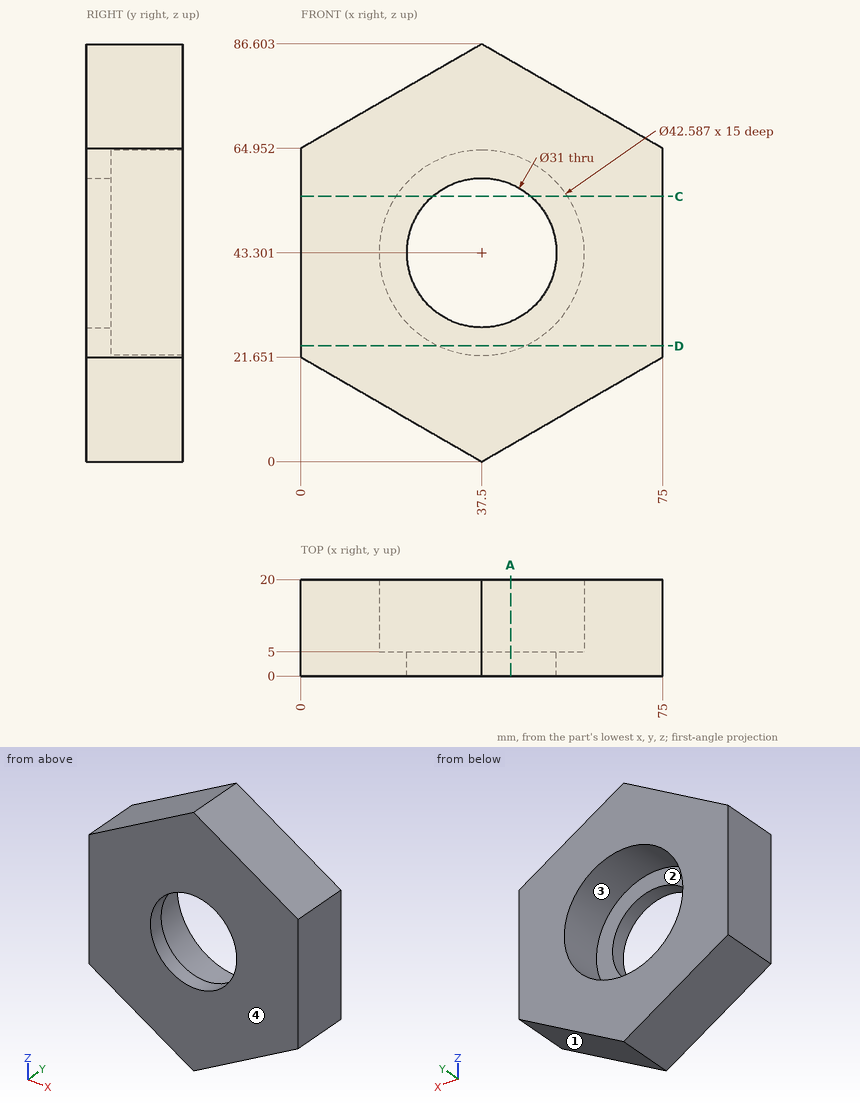
Design review of the part shown in the three views and the two pictorial views. Dimensions are in mm from the part's minimum x, y and z. Coordinates: 2 decimals unless noted, no trailing zeros. Loops run counter-clockwise (first coordinate to the right, second up) from the corner with the lowest first, then second, coordinate; pieces in that order, holes last. Notation, with made-up numbers: (-20.75, 79.25) - (37.25, 79.25) arc R24 cw to (37.25, 113.25) - close; hole circle Ø3 at (40.25, 27). An arc over 180 degrees is marked (long way). Use a Markdown table: item, result. Add a question column.
Item 1: Mouldability with a two-part tool opening along Z and no side actions: class the marked faces 1, 2, 3 and 4 as pulls with the +Z half, pulls with the -Z half, needs draft (parallel to the pull), parting line crosses it, or undercut.
Item 2: For line 1 (Z direction, x = 20, y = 9.5) (1 decimal); line 2 (Z direction, x = 33, y = 7) (1 decimal); line 3 (X direction, y = 8.25, z = 26) (1 decimal), list the stretches that pass through material, from the lowest coordinate up.
Item 3: Insertion check: pin 1 Ø1 at (x, y) = (30, 10) entering from +Z; pin 2 Ø1.5 at (x, y) = (35.5, 10.5) entering from -Z; pin 3 Ø21.5 at (x, z) = (43, 49.5) entering from +Y. Each pin has a flat end and moves straight along its axis. Give the tip position at first contact, or say it passes through.
Item 4: We need section D-D (z = 24). Give the boundary of the cut face in (x, y), and give its area (3 significant figures).
Item 5: We need section C-C (z = 55). Give the boundary of the cut face in (x, y).
Item 6: We need section A-A (x = 43.5). Give the boundary of the cut face in (y, z), and give its area (3 significant figures).
Results list:
| question | item | result |
|---|---|---|
| 1 | face 1 | pulls with the -Z half |
| 1 | face 2 | undercut |
| 1 | face 3 | undercut |
| 1 | face 4 | needs draft |
| 2 | line 1 | z = 10.1 to 31.2, 55.4 to 76.5 |
| 2 | line 2 | z = 2.6 to 22.5, 64.1 to 84 |
| 2 | line 3 | x = 0 to 25.1, 49.9 to 75 |
| 3 | pin 1 | stops at z = 82.56 |
| 3 | pin 2 | stops at z = 0.72 |
| 3 | pin 3 | stops at y = 5 |
| 4 | outline | (0, 0) - (75, 0) - (75, 20) - (46.49, 20) - (46.49, 5) - (28.51, 5) - (28.51, 20) - (0, 20) - close |
| 4 | area | 1,230 mm^2 |
| 5 | outline | (0, 0) - (27.33, 0) - (27.33, 5) - (19.71, 5) - (19.71, 20) - (0, 20) - close; (47.67, 0) - (75, 0) - (75, 20) - (55.29, 20) - (55.29, 5) - (47.67, 5) - close |
| 6 | outline | (0, 3.46) - (20, 3.46) - (20, 22.87) - (5, 22.87) - (5, 29.01) - (0, 29.01) - close; (0, 57.59) - (5, 57.59) - (5, 63.73) - (20, 63.73) - (20, 83.14) - (0, 83.14) - close |
| 6 | area | 838 mm^2 |
